```python
from build123d import *

# Parameters (mm, degrees)
F1_DEPTH = 8
F2_W     = 10.141368
F2_H     = 15
F3_DEPTH = 2


with BuildPart() as f1:
    # F0 (on Top) → F1 (new body)
    with BuildSketch(Plane.XY):
        with BuildLine():
            ThreePointArc((-4.451161, 2.035714), (-0.5, 0), (-4.451161, -2.035714))
            ThreePointArc((-4.451161, -2.035714), (-5.845911, -2.269536), (-5.612089, -3.664286))
            ThreePointArc((-5.612089, -3.664286), (-4.724749, -4.15635), (-3.749722, -4.437107))
            Line((-3.749722, -4.437107), (0, -5.070684))
            Line((0, -5.070684), (0, 5.070684))
            Line((0, 5.070684), (-3.749722, 4.437107))
            ThreePointArc((-3.749722, 4.437107), (-4.724749, 4.15635), (-5.612089, 3.664286))
            ThreePointArc((-5.612089, 3.664286), (-5.845911, 2.269536), (-4.451161, 2.035714))
        make_face()
    extrude(amount=F1_DEPTH)

    # F2 (on face) → F3 (join)
    with BuildSketch(Plane.YZ):
        with Locations((0, 4)):
            Rectangle(F2_W, F2_H)
    extrude(amount=F3_DEPTH)


solid = f1.part
```
For this review, take the finished solid that the model builds, in its own axes (mm). A direction names the side the tool comes from. Coordinates: 2 decimals unless noted, no trailing zeros. Loops run counter-clockwise (first coordinate to the right, second up) from the corner with the lowest first, then second, coordinate; pieces in that order, holes last.
1. For faces 1 (the flat face through (0, 0, -2)), 2 (the flat face through (0, 0, 10)), 3 (the cylindrical face through (-0.5, 0.1, 3.9)), list the 3-axis set-ups (+Z, -Z, +X, -X, +Y, -Y) from which the entire face can be reached by the end or side of a thin tool; tool diameter is ignored.
2. Add section A-A, the plane y = -2.85. Give the boundary of the cut face in (x, z).
3. Mouldability with a two-part tool opening along X and no side actions: class faces 4 (the cylindrical face through (-5.86, 2.29, 3.94)), 5 (the flat face through (-1.85, 4.76, 3.94)), 6 (the flat face through (-0.4, -1.1, 0)) as +X half, -X half, draft (parallel to the pull), parting line (faces both ways), or undercut.
4. Add section B-B, the plane x = -3. Give the boundary of the cut face in (y, z), then the cut area to 3 significant figures.
5. Insertion check: P1, Ø1.5, axis at y = 1, z = 7.5, coming from the -X side; P2, Ø1.8, axis at y = 2, z = 10, coming from the -X side; P3, Ø4, axis at x = -5, z = 6.5, coming from the +Y side; P4, Ø3, axis at x = -3, y = 0, coming from the +Z side. Each pin has a flat end and moves straight along its axis. Give the tip position at first contact, or say it passes through.
6. Add section D-D, the plane y = 0. Give the boundary of the cut face in (x, z).
7. For line 1 (X direction, y = 2, z = -0.25); line 2 (X direction, y = 0, z = 6.25); line 3 (Y direction, x = -1, z = 3.5), list the stretches that pass through material, from the lowest coordinate up.
8. Add section C-C, the plane z = 4. Give the boundary of the cut face in (x, y).
Result:
1. face 1: -Z, -X, +Y, -Y
1. face 2: +Z, -X, +Y, -Y
1. face 3: +Z, -Z
2. outline: (-6.03, 0) - (0, 0) - (0, -3.5) - (2, -3.5) - (2, 11.5) - (0, 11.5) - (0, 8) - (-6.03, 8) - close
3. face 4: undercut
3. face 5: -X half
3. face 6: draft
4. outline: (-4.56, 0) - (-2.5, 0) - (-2.5, 8) - (-4.56, 8) - close; (2.5, 0) - (4.56, 0) - (4.56, 8) - (2.5, 8) - close
4. area: 33.0 mm2
5. P1: stops at x = -1.21
5. P2: stops at x = 0
5. P3: stops at y = 4.56
5. P4: passes through
6. outline: (-0.5, 0) - (0, 0) - (0, -3.5) - (2, -3.5) - (2, 11.5) - (0, 11.5) - (0, 8) - (-0.5, 8) - close
7. line 1: x = 0 to 2
7. line 2: x = -0.5 to 2
7. line 3: y = -4.9 to -1.5, 1.5 to 4.9
8. outline: (-5.61, -3.66) arc R4.5 ccw to (-3.75, -4.44) - (0, -5.07) - (2, -5.07) - (2, 5.07) - (0, 5.07) - (-3.75, 4.44) arc R4.5 ccw to (-5.61, 3.66) arc R1 ccw to (-4.45, 2.04) arc R2.5 cw (long way) to (-4.45, -2.04) arc R1 ccw to start
